```python
from build123d import *

# Parameters (mm, degrees)
SKETCH2_R           = 2.5
BOSS_EXTRUDE1_DEPTH = 3
CUT_EXTRUDE1_DEPTH  = 4
SKETCH4_R           = 4
CUT_EXTRUDE2_DEPTH  = 5


with BuildPart() as part:
    # Sketch2 → Boss-Extrude1 (new body)
    with BuildSketch(Plane(origin=(0, 0, 0), x_dir=(1, 0, 0), z_dir=(0, 1, 0))):
        Polygon((-80, -37.5), (-80, -56.28), (98.09, -56.28), (98.09, 47.5), (-80, 47.5), align=None)
        with Locations((-70, -37.5)):
            Circle(SKETCH2_R, mode=Mode.SUBTRACT)
        with Locations((-70, 37.5)):
            Circle(SKETCH2_R, mode=Mode.SUBTRACT)
        with Locations((70, 37.5)):
            Circle(SKETCH2_R, mode=Mode.SUBTRACT)
        with Locations((70, -37.5)):
            Circle(SKETCH2_R, mode=Mode.SUBTRACT)
    extrude(amount=BOSS_EXTRUDE1_DEPTH)

    # Sketch3 → Cut-Extrude1 (cut, through all)
    with BuildSketch(Plane(origin=(0, 3, 0), x_dir=(1, 0, 0), z_dir=(0, 1, 0))):
        Polygon((98.09, -56.28), (94.09, -56.28), (98.09, -52.28), align=None)
    extrude(amount=-CUT_EXTRUDE1_DEPTH, mode=Mode.SUBTRACT)

    # Sketch4 → Cut-Extrude2 (cut)
    with BuildSketch(Plane(origin=(0, 3, 0), x_dir=(1, 0, 0), z_dir=(0, 1, 0))):
        with Locations((-1.66, 21.61)):
            Circle(SKETCH4_R)
        with Locations((-1.66, -30.39)):
            Circle(SKETCH4_R)
    extrude(amount=-CUT_EXTRUDE2_DEPTH, mode=Mode.SUBTRACT)


solid = part.part
```
Geometry check sheet. Reference: the model listing, model coordinates, mm. Give positions to 0.01 mm unless a question says otherwise; leave off trailing zeros. Write each loop counter-clockwise with the first axis right and the second up, starting at its lowest first coordinate (ties: lowest second). Pieces come first, ordered by that corner, then holes.
1) Release check for a two-part mould opening along X. For faces 1 (the flat face through (8, 0, 4)), 2 (the flat face through (96.06, 1.52, 54.31)), 3 (the cylindrical face through (-70.54, 1.48, -35.06)) record: pulls with the +X half, pulls with the -X half, needs draft (parallel to the pull), parting line crosses it, or undercut.
2) Section check A-A, the plane x = -1.66. Record the boundary of the cut face in (y, z), and give its area (3 significant figures).
3) Material ranges on L1, parallel to Z at x = -1.66, y = 1.45; L2, parallel to Z at x = 70, y = 2.05; L3, parallel to X at y = 1.35, z = 37.5, recorded low to high.
4) Section check C-C, the plane x = 70. Record the boundary of the cut face in (y, z), and give its area (3 significant figures).
5) Section check B-B, the plane z = 30.39. Record the boundary of the cut face in (x, y).
Computed:
1. face 1: needs draft
1. face 2: pulls with the +X half
1. face 3: undercut
2. outline: (0, -47.5) - (3, -47.5) - (3, -25.61) - (0, -25.61) - close; (0, -17.61) - (3, -17.61) - (3, 26.39) - (0, 26.39) - close; (0, 34.39) - (3, 34.39) - (3, 56.28) - (0, 56.28) - close
2. area: 263 mm2
3. L1: z = -47.5 to -25.61, -17.61 to 26.39, 34.39 to 56.28
3. L2: z = -47.5 to -40, -35 to 35, 40 to 56.28
3. L3: x = -80 to -72.5, -67.5 to 67.5, 72.5 to 98.09
4. outline: (0, -47.5) - (3, -47.5) - (3, -40) - (0, -40) - close; (0, -35) - (3, -35) - (3, 35) - (0, 35) - close; (0, 40) - (3, 40) - (3, 56.28) - (0, 56.28) - close
4. area: 281 mm2
5. outline: (-80, 0) - (-5.66, 0) - (-5.66, 3) - (-80, 3) - close; (2.34, 0) - (98.09, 0) - (98.09, 3) - (2.34, 3) - close
